Source: CAD feature listing. Evaluate the final solid. Frame: model axes, mm. Face numbers are marked on the shaded views. A direction names the side the tool comes from. Round coordinates to 2 decimals unless told otherwise and drop trailing zeros. Order: outer loops, then holes, each group sorted by start corner. A loop starts at its lowest first (then second) coordinate and runs counter-clockwise, first axis right, second up. Notation, with made-up numbers: (-19, 56.5) -> (30, 56.5) arc R38 ccw to (30, 94.5) -> close; hole circle Ø10 at (19.5, 56.5). An arc over 180 degrees is marked (long way). Answer as CSV lines item,"result". Start each with the question number.
(1) Section query B-B (z = 1.1). Output: boundary loops of the cut face in (x, y).
(2) Line query: line 1 along Z through (x, y) = (6.5, 2.85); line 2 along Z through (x, y) = (4.75, 3.05); line 3 along X through (y, z) = (3.5, 3.8). Output: solid intervals per line, ascending. Write a range as from..to.
(3) Section query A-A (x = 4.25). Output: boundary loops of the cut face in (y, z).
(4) Section query D-D (x = 9.25). Output: boundary loops of the cut face in (y, z).
(5) Section query C-C (y = 4.6). Output: boundary loops of the cut face in (x, z), plus the area to 3 significant figures.
(6) Pull-direction query (X, two-part tool) for the marked faces 1, 2 and 3; classes: +X half, -X half, draft (parallel to the pull), parting line (faces both ways), or undercut.
(7) Set-up query: the marked faces 4 and 5. Return all of +Z, -Z, +X, -X, +Y, -Y with unobstructed straight access to the full face (end or side cutting, diameter ignored); none if empty.
(8) Contact query for flat-ended pins moving along their axis: P1, Ø1.5, axis at x = 3.5, y = 1.5, coming from the +Z side; P2, Ø3, axis at y = 3.5, z = 3.5, coming from the -X side. Output: stop coordinate, or through.
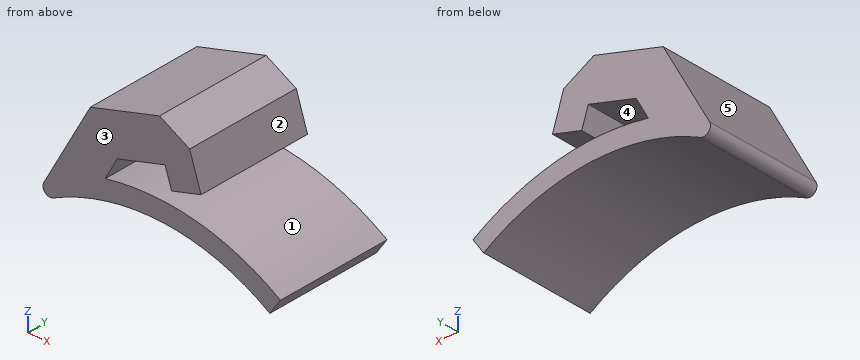
```python
from build123d import *

# Parameters (mm, degrees)
EXTRUDE_1_DEPTH = 5
CHAMFER_1_SIZE  = 1
CHAMFER_1_SIZE2 = 1.032395136


with BuildPart() as part:
    # Эскиз1 → Бобышка-Вытянуть1 (new body)
    with BuildSketch(Plane(origin=(0, 0, 0), x_dir=(1, 0, 0), z_dir=(0, 1, 0))):
        with BuildLine():
            Line((2.5, -4.5), (6.395063253, -5.64))
            Line((6.395063253, -5.64), (7.2, -3.175018115))
            Line((7.2, -3.175018115), (5.952339772, -2.809855198))
            Line((5.952339772, -2.809855198), (5.675364666, -3.658044352))
            Line((5.675364666, -3.658044352), (3.647199382, -3.06444464))
            Line((3.647199382, -3.06444464), (3.126833621, -2.12778627))
            ThreePointArc((3.126833621, -2.12778627), (6.994242164, -2.125926125), (10.57111662, -0.655272725))
            Line((10.57111662, -0.655272725), (10.119998501, 0.005508219))
            ThreePointArc((10.119998501, 0.005508219), (5.594481852, -1.5), (0.923871938, -0.534464416))
            ThreePointArc((0.923871938, -0.534464416), (0.572572084, -0.594660683), (0.526733755, -0.948120759))
            Line((0.526733755, -0.948120759), (2.5, -4.5))
        make_face()
    extrude(amount=EXTRUDE_1_DEPTH)

    # Фаска1
    chamfer_1_edges = [part.edges().sort_by_distance(p)[0] for p in [
        (6.395063253, 2.5, 5.64),
    ]]
    chamfer_1_side = [part.faces().sort_by_distance(p)[0] for p in [
        (4.447531626, 2.5, 5.07),
    ]]
    chamfer(chamfer_1_edges, length=CHAMFER_1_SIZE, length2=CHAMFER_1_SIZE2, reference=chamfer_1_side[0])


solid = part.part
```
Answer block:
1,outline,"(0.61, 0) -> (2.32, 0) -> (2.32, 5) -> (0.61, 5) -> close; (7.79, 0) -> (9.83, 0) -> (9.83, 5) -> (7.79, 5) -> close"
2,line 1,"1.4..2.21, 2.97..4.78"
2,line 2,"1.51..2.31, 3.39..5.16"
2,line 3,"2.11..7"
3,outline,"(0, 1.48) -> (5, 1.48) -> (5, 2.28) -> (0, 2.28) -> close; (0, 3.24) -> (5, 3.24) -> (5, 5.01) -> (0, 5.01) -> close"
4,outline,"(0, 0.5) -> (5, 0.5) -> (5, 1.39) -> (0, 1.39) -> close"
5,outline,"(0.53, 0.95) arc R0.3 ccw to (0.92, 0.53) arc R9.19 cw to (10.12, -0.01) -> (10.57, 0.66) arc R9.99 ccw to (3.13, 2.13) -> (3.65, 3.06) -> (5.68, 3.66) -> (5.95, 2.81) -> (7.2, 3.18) -> (6.72, 4.66) -> (5.44, 5.36) -> (2.5, 4.5) -> close"
5,area,"19.0 mm2"
6,face 1,"undercut"
6,face 2,"+X half"
6,face 3,"draft"
7,face 4,"+Y, -Y"
7,face 5,"+Z, -X, +Y, -Y"
8,P1,"z = 5.01"
8,P2,"x = 1.11"
